```python
from build123d import *

# Parameters (mm, degrees)
SKETCH1_R           = 1.1049
BOSS_EXTRUDE1_DEPTH = 1.5875


with BuildPart() as part:
    # Sketch1 → Boss-Extrude1 (new body)
    with BuildSketch(Plane.XY):
        with BuildLine():
            Line((-7.084965338, 4.8768), (-17.181244816, 4.8768))
            ThreePointArc((-17.181244816, 4.8768), (-15.375234721, 9.087381854), (-12.557442768, 12.699959952))
            Line((-12.557442768, 12.699959952), (-14.138046409, 14.773078207))
            ThreePointArc((-14.138046409, 14.773078207), (-13.706164911, 17.976993058), (-10.502250061, 17.54511156))
            Line((-10.502250061, 17.54511156), (-8.92164642, 15.471993305))
            ThreePointArc((-8.92164642, 15.471993305), (2.385909574, 17.699880993), (12.699959952, 12.557442768))
            Line((12.699959952, 12.557442768), (14.773078207, 14.138046409))
            ThreePointArc((14.773078207, 14.138046409), (17.976993058, 13.706164911), (17.54511156, 10.502250061))
            Line((17.54511156, 10.502250061), (15.471993305, 8.92164642))
            ThreePointArc((15.471993305, 8.92164642), (16.316677959, 7.26253207), (16.984058744, 5.5245))
            Line((16.984058744, 5.5245), (16.984058744, -5.5245))
            ThreePointArc((16.984058744, -5.5245), (10.454687446, -14.480257667), (-0.100774867, -17.859680739))
            Line((-0.100774867, -17.859680739), (-0.449035291, -20.443252268))
            ThreePointArc((-0.449035291, -20.443252268), (-3.019931544, -22.40337585), (-4.980055125, -19.832479597))
            Line((-4.980055125, -19.832479597), (-4.631794702, -17.248908067))
            ThreePointArc((-4.631794702, -17.248908067), (-12.386896286, -12.866357374), (-17.060660873, -5.2832))
            Line((-17.060660873, -5.2832), (-7.084965338, -5.2832))
            Line((-7.084965338, -5.2832), (-7.084965338, 4.8768))
        make_face()
        with Locations((-2.714545208, -20.137865932)):
            Circle(SKETCH1_R, mode=Mode.SUBTRACT)
        with Locations((-12.320148235, 16.159094884)):
            Circle(SKETCH1_R, mode=Mode.SUBTRACT)
        with Locations((16.159094884, 12.320148235)):
            Circle(SKETCH1_R, mode=Mode.SUBTRACT)
    extrude(amount=BOSS_EXTRUDE1_DEPTH)


solid = part.part
```
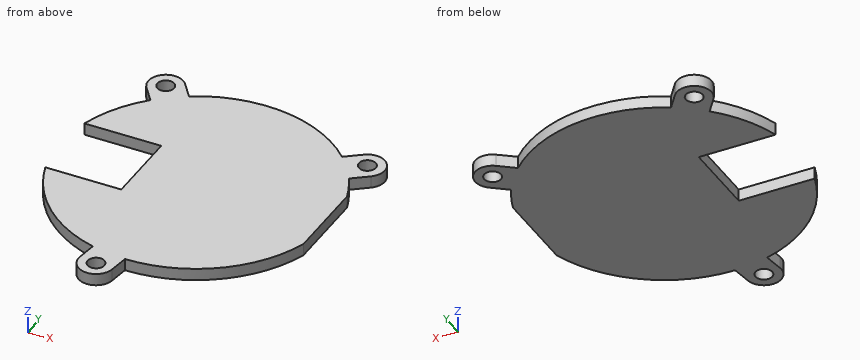
Design review of the part built by this model. Coordinates are the model's own, in mm. Give positions to 0.01 mm unless a question says otherwise; leave off trailing zeros. Write each loop counter-clockwise with the first axis right and the second up, starting at its lowest first coordinate (ties: lowest second). Pieces come first, ordered by that corner, then holes.
(1) Add section B-B (x = -2.5). Give the boundary of the cut face in (y, z), and give its area (3 significant figures).
Checked values:
outline: (-22.41, 0) - (-21.22, 0) - (-21.22, 1.59) - (-22.41, 1.59) - close; (-19.05, 0) - (17.68, 0) - (17.68, 1.59) - (-19.05, 1.59) - close
area: 60.2 mm2
(2) Clearance check with flat-ended pins moving along their axes: pin 1 Ø3 at (x, y) = (-12.5, -17) entering from -Z; pin 2 Ø0.8 at (y, z) = (-1, 1) entering from -X. State where each tip first meets the part, or that it passes through.
Checked values:
pin 1: passes through
pin 2: stops at x = -7.08
(3) Add section A-A (z = 0.95). Give the boundary of the cut face in (x, y).
Checked values:
outline: (-17.18, 4.88) - (-7.08, 4.88) - (-7.08, -5.28) - (-17.06, -5.28) arc R17.86 ccw to (-4.63, -17.25) - (-4.98, -19.83) arc R2.29 ccw to (-0.45, -20.44) - (-0.1, -17.86) arc R17.86 ccw to (16.98, -5.52) - (16.98, 5.52) arc R17.86 ccw to (15.47, 8.92) - (17.55, 10.5) arc R2.29 ccw to (14.77, 14.14) - (12.7, 12.56) arc R17.86 ccw to (-8.92, 15.47) - (-10.5, 17.55) arc R2.29 ccw to (-14.14, 14.77) - (-12.56, 12.7) arc R17.86 ccw to start; hole circle Ø2.21 at (-12.32, 16.16); hole circle Ø2.21 at (-2.71, -20.14); hole circle Ø2.21 at (16.16, 12.32)
(4) Add section C-C (y = -3). Give the boundary of the cut face in (x, z).
Checked values:
outline: (-7.08, 0) - (16.98, 0) - (16.98, 1.59) - (-7.08, 1.59) - close
(5) Wall thickness on line 1 along Y through (x, z) = (0.5, 0.65); line 2 along Y through (x, z) = (-13.5, 1.4); line 3 along X through (y, z) = (4, 1): over which ranges is each line inside the solid? List them lowest first.
Checked values:
line 1: y = -17.85 to 17.85
line 2: y = -11.69 to -5.28, 4.88 to 11.69, 13.94 to 18.12
line 3: x = -7.08 to 16.98
(6) Add section D-D (x = 7). Give the boundary of the cut face in (y, z).
Checked values:
outline: (-16.43, 0) - (16.43, 0) - (16.43, 1.59) - (-16.43, 1.59) - close
